Read the model definition and answer for the solid it produces. Units are mm, in the model's axes. A direction names the side the tool comes from. Round coordinates to 2 decimals unless told otherwise and drop trailing zeros. Order: outer loops, then holes, each group sorted by start corner. A loop starts at its lowest first (then second) coordinate and runs counter-clockwise, first axis right, second up. Notation, with made-up numbers: (59.25, 25.25) -> (93.25, 25.25) arc R24 ccw to (93.25, 59.25) -> close; hole circle Ø8 at (65, 18.5). An arc over 180 degrees is marked (long way). One line per item, written item: value. Start each with the question number.
1. The mould has two halves that part along Z. Classify faces 3 (the face through (36, 1, -1)), 4 (the face through (-35, 1, -43)), 5 (the face through (26, 1, 0)), 6 (the face through (35, 1, 43)): released by +Z, released by -Z, zero draft, split by the parting line, or undercut.
2. Section B-B (z = -4.5) is taken. Give the vertices of the cut face in (x, y).
3. Section A-A (x = 14) is taken. Give the vertices of the cut face in (y, z).
4. Section C-C (y = 1.45) is taken. State how many separate pieces and enclosed holes the cut face has, then the cut area to 3 significant figures.
5. For faces 1 (the face through (33, 0, -1)), 2 (the face through (0, 1, -35)), determine the directions among +Z, -Z, +X, -X, +Y, -Y from which every point of the face is accessible in a straight line to the end or side of a thin tool.
6. Consider line 1 (Z direction, x = 31, y = 1.8); line 2 (X direction, y = 0.55, z = 38); line 3 (X direction, y = 1.7, z = 40). Determine where each line is inside the solid, lowest interval first.
7. A flat-ended cylindrical pin translates along its axis: pin 1 Ø4 at (x, z) = (31, -40) entering from +Y. Find the tip coordinate at first contact, or state that the pin passes through.
from build123d import *

# Parameters (mm, degrees)
SKETCH_1_R      = 1.5
SKETCH_1_W      = 52
SKETCH_1_H      = 70
EXTRUDE_1_DEPTH = 2.4
FILLET_1_R      = 5


with BuildPart() as part:
    # 草圖1 → 填料-伸長1 (new body)
    with BuildSketch(Plane(origin=(0, 0, 0), x_dir=(1, 0, 0), z_dir=(0, 1, 0))):
        with BuildLine():
            Line((-31, 45), (31, 45))
            ThreePointArc((31, 45), (34.535533906, 43.535533906), (36, 40))
            Line((36, 40), (36, -40))
            ThreePointArc((36, -40), (34.535533906, -43.535533906), (31, -45))
            Line((31, -45), (-31, -45))
            ThreePointArc((-31, -45), (-34.535533906, -43.535533906), (-36, -40))
            Line((-36, -40), (-36, 40))
            ThreePointArc((-36, 40), (-34.535533906, 43.535533906), (-31, 45))
        make_face()
        with Locations((-26, 38)):
            Circle(SKETCH_1_R, mode=Mode.SUBTRACT)
        with Locations((26, 38)):
            Circle(SKETCH_1_R, mode=Mode.SUBTRACT)
        with Locations((26, -38)):
            Circle(SKETCH_1_R, mode=Mode.SUBTRACT)
        with Locations((-26, -38)):
            Circle(SKETCH_1_R, mode=Mode.SUBTRACT)
        with Locations((-31, 40)):
            Circle(SKETCH_1_R, mode=Mode.SUBTRACT)
        with Locations((31, 40)):
            Circle(SKETCH_1_R, mode=Mode.SUBTRACT)
        with Locations((-31, -40)):
            Circle(SKETCH_1_R, mode=Mode.SUBTRACT)
        with Locations((31, -40)):
            Circle(SKETCH_1_R, mode=Mode.SUBTRACT)
        Rectangle(SKETCH_1_W, SKETCH_1_H, mode=Mode.SUBTRACT)
    extrude(amount=EXTRUDE_1_DEPTH)

    # 圓角1
    fillet_1_edges = [part.edges().sort_by_distance(p)[0] for p in [
        (26, 1.2, -35),
        (-26, 1.2, -35),
        (-26, 1.2, 35),
        (26, 1.2, 35),
    ]]
    fillet(fillet_1_edges, radius=FILLET_1_R)


solid = part.part
Answer:
1. face 3: zero draft
1. face 4: released by -Z
1. face 5: undercut
1. face 6: released by +Z
2. outline: (-36, 0) -> (-26, 0) -> (-26, 2.4) -> (-36, 2.4) -> close; (26, 0) -> (36, 0) -> (36, 2.4) -> (26, 2.4) -> close
3. outline: (0, -45) -> (2.4, -45) -> (2.4, -35) -> (0, -35) -> close; (0, 35) -> (2.4, 35) -> (2.4, 45) -> (0, 45) -> close
4. separate pieces: 1
4. enclosed holes: 9
4. area: 2,780 mm^2
5. face 1: +Z, -Z, +X, -X, -Y
5. face 2: +Y, -Y
6. line 1: -45 to -41.5, -38.5 to 38.5, 41.5 to 45
6. line 2: -36 to -27.5, -24.5 to 24.5, 27.5 to 36
6. line 3: -36 to -32.5, -29.5 to 29.5, 32.5 to 36
7. pin 1: y = 2.4
